Part model, mm, in its own coordinate system. A direction names the side the tool comes from. Coordinates: 2 decimals unless noted, no trailing zeros. Loops run counter-clockwise (first coordinate to the right, second up) from the corner with the lowest first, then second, coordinate; pieces in that order, holes last. Notation, with made-up numbers: (21.25, 10) -> (76.25, 10) arc R13 ccw to (76.25, 26) -> close; hole circle Ø2 at (-20.5, 87). An arc over 180 degrees is marked (long way). Use one line per item in the form item = value. Start each with the question number.
(1) Band-saw the part on B-B on y = -25. Give the cut face in (x, z).
(2) Band-saw the part on D-D on x = 1. Give the cut face in (y, z).
(3) Drill centre lines: L1, parallel to X at y = 0, z = 2.3; L2, parallel to Y at x = -11, z = 3.3; L3, parallel to Y at x = 0.5, z = 2.5. Where is each one in solid material? Low to high. Write a range as [from, to].
(4) Mould opens along Y. For faces 1 (the flat face through (0, 7, 0)), 2 (the flat face through (-4.261, -5.634, 2.613)), 3 (the cylindrical face through (14.14, 29.1, 2.61)) say: +Y half, -Y half, draft (parallel to the pull), parting line (faces both ways), or undercut.
(5) 3-axis set-ups, long thin cutter, end or side, ignore diameter. For faces 4 (the flat face through (15, 23, 3)), 5 (the flat face through (-4.301, 5.644, 2.613)), 6 (the cylindrical face through (-14.1, 29.14, 2.61)), 7 (the flat face through (0, 30, 3)), 8 (the flat face through (-15, -23, 3)): which of +Z, -Z, +X, -X, +Y, -Y reach the whole face in a straight line?
(6) Pin check, flat tips, straight feed: P1, Ø0.8, axis at x = 17.5, z = 2, coming from the +Y side; P2, Ø1.6, axis at y = 22, z = 3, coming from the +X side; P3, Ø2.5, axis at y = 24, z = 4, coming from the -X side. Stop position of each tip, or through.
(7) Band-saw the part on C-C on z = 2.3. Count the separate pieces of the cut face and the enclosed holes in it, then the cut area to 3 significant figures.
(8) Band-saw the part on A-A on x = -11. Give the cut face in (y, z).
```python
from build123d import *

# Parameters (mm, degrees)
F0_R     = 2.5
F1_DEPTH = 5.3


with BuildPart() as f1:
    # F0 (on Top) → F1 (new body)
    with BuildSketch(Plane.XY):
        with BuildLine():
            Line((-12, -30), (12, -30))
            ThreePointArc((12, -30), (14.12132, -29.12132), (15, -27))
            Line((15, -27), (15, -19.5))
            ThreePointArc((15, -19.5), (15.585786, -18.085786), (17, -17.5))
            Line((17, -17.5), (18, -17.5))
            ThreePointArc((18, -17.5), (19.414214, -16.914214), (20, -15.5))
            Line((20, -15.5), (20, 15.5))
            ThreePointArc((20, 15.5), (19.414214, 16.914214), (18, 17.5))
            Line((18, 17.5), (17, 17.5))
            ThreePointArc((17, 17.5), (15.585786, 18.085786), (15, 19.5))
            Line((15, 19.5), (15, 27))
            ThreePointArc((15, 27), (14.12132, 29.12132), (12, 30))
            Line((12, 30), (-12, 30))
            ThreePointArc((-12, 30), (-14.12132, 29.12132), (-15, 27))
            Line((-15, 27), (-15, 19.5))
            ThreePointArc((-15, 19.5), (-15.585786, 18.085786), (-17, 17.5))
            Line((-17, 17.5), (-18, 17.5))
            ThreePointArc((-18, 17.5), (-19.414214, 16.914214), (-20, 15.5))
            Line((-20, 15.5), (-20, -15.5))
            ThreePointArc((-20, -15.5), (-19.414214, -16.914214), (-18, -17.5))
            Line((-18, -17.5), (-17, -17.5))
            ThreePointArc((-17, -17.5), (-15.585786, -18.085786), (-15, -19.5))
            Line((-15, -19.5), (-15, -27))
            ThreePointArc((-15, -27), (-14.12132, -29.12132), (-12, -30))
        make_face()
        with Locations((0, -25)):
            Circle(F0_R, mode=Mode.SUBTRACT)
        with BuildLine():
            ThreePointArc((-5.708497, -6), (-19, 0), (-5.708497, 6))
            Line((-5.708497, 6), (-2.854249, 5.277619))
            ThreePointArc((-2.854249, 5.277619), (-1.472122, 5.816602), (0, 6))
            ThreePointArc((0, 6), (6, 0), (0, -6))
            ThreePointArc((0, -6), (-1.472122, -5.816602), (-2.854249, -5.277619))
            Line((-2.854249, -5.277619), (-5.708497, -6))
        make_face(mode=Mode.SUBTRACT)
        with Locations((0, 25)):
            Circle(F0_R, mode=Mode.SUBTRACT)
    extrude(amount=F1_DEPTH)


solid = f1.part
```
A:
q1.outline = (-15, 0) -> (-2.5, 0) -> (-2.5, 5.3) -> (-15, 5.3) -> close; (2.5, 0) -> (15, 0) -> (15, 5.3) -> (2.5, 5.3) -> close
q2.outline = (-30, 0) -> (-27.29, 0) -> (-27.29, 5.3) -> (-30, 5.3) -> close; (-22.71, 0) -> (-5.92, 0) -> (-5.92, 5.3) -> (-22.71, 5.3) -> close; (5.92, 0) -> (22.71, 0) -> (22.71, 5.3) -> (5.92, 5.3) -> close; (27.29, 0) -> (30, 0) -> (30, 5.3) -> (27.29, 5.3) -> close
q3.L1 = [-20, -19], [6, 20]
q3.L2 = [-30, -8], [8, 30]
q3.L3 = [-30, -27.45], [-22.55, -5.98], [5.98, 22.55], [27.45, 30]
q4.face_1 = draft
q4.face_2 = undercut
q4.face_3 = +Y half
q5.face_4 = +Z, -Z, +X, +Y
q5.face_5 = +Z, -Z
q5.face_6 = +Z, -Z, -X, +Y
q5.face_7 = +Z, -Z, +X, -X, +Y
q5.face_8 = +Z, -Z, -X, -Y
q6.P1 = 17.5
q6.P2 = 15
q6.P3 = -15
q7.separate_pieces = 1
q7.enclosed_holes = 3
q7.area = 1,800 mm²
q8.outline = (-30, 0) -> (-8, 0) -> (-8, 5.3) -> (-30, 5.3) -> close; (8, 0) -> (30, 0) -> (30, 5.3) -> (8, 5.3) -> close
